Source: CAD feature listing. Evaluate the final solid. Frame: model axes, mm. Round coordinates to 2 decimals unless told otherwise and drop trailing zeros. Order: outer loops, then holes, each group sorted by start corner. A loop starts at its lowest first (then second) coordinate and runs counter-clockwise, first axis right, second up. Notation, with made-up numbers: M -35.5,-8 L -20.5,-8 A22 ccw -20.5,12 Z; hole C 69.5,39 d4. An arc over 180 degrees is marked long. Answer as CSV lines item,"result". Start each with the question number.
Item 1: Section query A-A on y = 8. Return the cut outline in (x, z), plus the area to 3 significant figures.
Item 2: Section query D-D on z = -12.5. Return the cut outline in (x, y).
Item 3: First-contact query: P1, Ø3, axis at x = 37.5, y = 2.5, coming from the +Z side; P2, Ø9, axis at x = 47, y = -1.5, coming from the -Z side; P3, Ø9, axis at x = 36, z = -3, coming from the +Y side; P4, Ø3.5, axis at y = 13, z = -12.5, coming from the -X side. Flat tips, straight axial feed; report the tip coordinate or a pass-through.
Item 4: Pull-direction query (X, two-part tool) for faces 1 (the face through (109, 8, 0)), 2 (the face through (107, 17, -16)), 3 (the face through (54, 0, 9)); classes: +X half, -X half, draft (parallel to the pull), parting line (faces both ways), or undercut.
Item 5: Line query: line 1 (Z direction, x = 3.5, y = -13); line 2 (Y direction, x = 106, z = -12.5); line 3 (X direction, y = -4.5, z = 10). Output: solid intervals per line, ascending. Write a range as [from, to].
Item 6: Section query B-B on z = -6.5. Return the cut outline in (x, y), plus the area to 3 significant figures.
Item 7: Section query C-C on x = 13.5. Return the cut outline in (y, z).
from build123d import *

# Parameters (mm, degrees)
SKETCH_1_W                  = 35
SKETCH_1_H                  = 35
SKETCH_1_W_2                = 16
SKETCH_1_H_2                = 8
EXTRUDE_1_DEPTH             = 4.5
CHAMFER_1_SIZE              = 2
SKETCH_4_W                  = 18
SKETCH_4_H                  = 10
SKETCH_4_W_2                = 16
SKETCH_4_H_2                = 8
EXTRUDE_2_DEPTH             = 100
SKETCH_5_W                  = 35
SKETCH_5_H                  = 35
SKETCH_5_W_2                = 16
SKETCH_5_H_2                = 8
EXTRUDE_3_DEPTH             = 4.5
CHAMFER_2_SIZE              = 2
HOLE_WIZARD_4_5_4_5_2_D     = 4.5
PATTERN_LINEAR_1_COUNT      = 2
PATTERN_LINEAR_1_PITCH      = 25
PATTERN_LINEAR_1_COUNT_DIR2 = 2
PATTERN_LINEAR_1_PITCH_DIR2 = 26


with BuildPart() as part:
    # Эскиз1 → Бобышка-Вытянуть1 (new body)
    with BuildSketch(Plane(origin=(0, 0, 0), x_dir=(0, 0, -1), z_dir=(1, 0, 0))):
        Rectangle(SKETCH_1_W, SKETCH_1_H)
        Rectangle(SKETCH_1_W_2, SKETCH_1_H_2, mode=Mode.SUBTRACT)
    extrude(amount=EXTRUDE_1_DEPTH)

    # Фаска1
    chamfer_1_edges = [part.edges().sort_by_distance(p)[0] for p in [
        (2.25, -17.5, -17.5),
        (2.25, -17.5, 17.5),
        (2.25, 17.5, 17.5),
        (2.25, 17.5, -17.5),
    ]]
    chamfer(chamfer_1_edges, length=CHAMFER_1_SIZE)

    # Эскиз4 → Бобышка-Вытянуть2 (add)
    with BuildSketch(Plane(origin=(4.5, 0, 0), x_dir=(0, 0, -1), z_dir=(1, 0, 0))):
        Rectangle(SKETCH_4_W, SKETCH_4_H)
        Rectangle(SKETCH_4_W_2, SKETCH_4_H_2, mode=Mode.SUBTRACT)
    extrude(amount=EXTRUDE_2_DEPTH)

    # Эскиз5 → Бобышка-Вытянуть3 (add)
    with BuildSketch(Plane(origin=(104.5, 0, 0), x_dir=(0, 0, -1), z_dir=(1, 0, 0))):
        Rectangle(SKETCH_5_W, SKETCH_5_H)
        Rectangle(SKETCH_5_W_2, SKETCH_5_H_2, mode=Mode.SUBTRACT)
    extrude(amount=EXTRUDE_3_DEPTH)

    # Фаска2
    chamfer_2_edges = [part.edges().sort_by_distance(p)[0] for p in [
        (106.75, -17.5, -17.5),
        (106.75, 17.5, -17.5),
        (106.75, 17.5, 17.5),
        (106.75, -17.5, 17.5),
    ]]
    chamfer(chamfer_2_edges, length=CHAMFER_2_SIZE)

    # Диаметр отверстия Ø4.5 (4.5)2 (through all)
    with Locations(Plane(origin=(0, 13, 12.5), x_dir=(0, 0, -1), z_dir=(-1, 0, 0))):
        with Locations((0, 0)):
            hole_wizard_4_5_4_5_2 = Hole(HOLE_WIZARD_4_5_4_5_2_D / 2)

    # Линейный массив1: Hole Wizard 4.5 _4.5_2 2 × 2
    with Locations(*[(0, -j * PATTERN_LINEAR_1_PITCH_DIR2, -i * PATTERN_LINEAR_1_PITCH) for i in range(PATTERN_LINEAR_1_COUNT) for j in range(PATTERN_LINEAR_1_COUNT_DIR2) if (i, j) != (0, 0)]):
        add(hole_wizard_4_5_4_5_2, mode=Mode.SUBTRACT)


solid = part.part
Results:
1,outline,"M 0,-17.5 L 4.5,-17.5 L 4.5,17.5 L 0,17.5 Z; M 104.5,-17.5 L 109,-17.5 L 109,17.5 L 104.5,17.5 Z"
1,area,"315 mm^2"
2,outline,"M 0,-17.5 L 4.5,-17.5 L 4.5,-15.25 L 0,-15.25 Z; M 0,-10.75 L 4.5,-10.75 L 4.5,10.75 L 0,10.75 Z; M 0,15.25 L 4.5,15.25 L 4.5,17.5 L 0,17.5 Z; M 104.5,-17.5 L 109,-17.5 L 109,-15.25 L 104.5,-15.25 Z; M 104.5,-10.75 L 109,-10.75 L 109,10.75 L 104.5,10.75 Z; M 104.5,15.25 L 109,15.25 L 109,17.5 L 104.5,17.5 Z"
3,P1,"z = 9"
3,P2,"z = -9"
3,P3,"y = 5"
3,P4,"through"
4,face 1,"+X half"
4,face 2,"draft"
4,face 3,"undercut"
5,line 1,"[-17.5, -14.75], [-10.25, 10.25], [14.75, 17.5]"
5,line 2,"[-17.5, -15.25], [-10.75, 10.75], [15.25, 17.5]"
5,line 3,"[0, 4.5], [104.5, 109]"
6,outline,"M 0,-17.5 L 4.5,-17.5 L 4.5,-5 L 104.5,-5 L 104.5,-17.5 L 109,-17.5 L 109,-4 L 0,-4 Z; M 0,4 L 109,4 L 109,17.5 L 104.5,17.5 L 104.5,5 L 4.5,5 L 4.5,17.5 L 0,17.5 Z"
6,area,"443 mm^2"
7,outline,"M -5,-9 L 5,-9 L 5,9 L -5,9 Z; hole M -4,-8 L 4,-8 L 4,8 L -4,8 Z"
